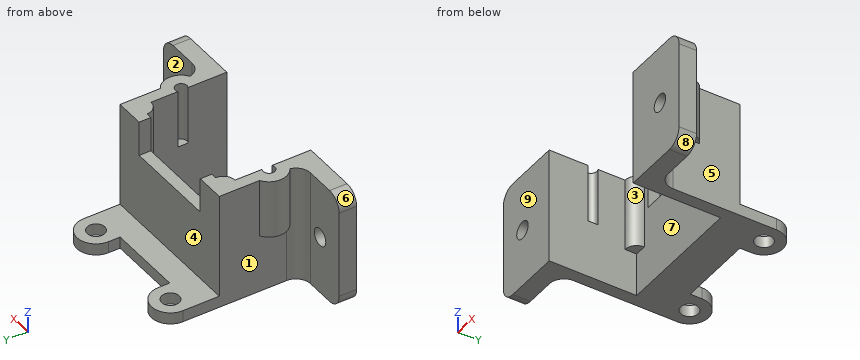
```python
from build123d import *

# Parameters (mm, degrees)
EXTRUDE_1_DEPTH     = 20
CUT_EXTRUDE_1_DEPTH = 20
EXTRUDE_2_DEPTH     = 12.5
SKETCH_4_W          = 4.208324297
SKETCH_4_H          = 5.852484321
SKETCH_4_W_2        = 6.809838445
SKETCH_4_H_2        = 5.603711631
CUT_EXTRUDE_2_DEPTH = 10
EXTRUDE_3_DEPTH     = 10
SKETCH_6_W          = 10
SKETCH_6_H          = 20
EXTRUDE_4_DEPTH     = 3
SKETCH_7_R          = 1.5
CUT_EXTRUDE_3_DEPTH = 3
FILLET_1_R          = 2.5
SKETCH_8_R          = 1.5
EXTRUDE_5_DEPTH     = 2


with BuildPart() as part:
    # 草图1 → 凸台-拉伸1 (new body)
    with BuildSketch(Plane.XY):
        with BuildLine():
            Line((-15.073529412, 6.665686275), (10.926470588, 6.665686275))
            Line((10.926470588, 6.665686275), (10.926470588, -0.236237514))
            ThreePointArc((10.926470588, -0.236237514), (12.426470588, -2.834313725), (10.926470588, -5.432389937))
            Line((10.926470588, -5.432389937), (10.926470588, -10.334313725))
            Line((10.926470588, -10.334313725), (8.926470588, -10.334313725))
            Line((8.926470588, -10.334313725), (8.926470588, -3.700339129))
            ThreePointArc((8.926470588, -3.700339129), (10.426470588, -2.834313725), (8.926470588, -1.968288322))
            Line((8.926470588, -1.968288322), (8.926470588, 4.665686275))
            Line((8.926470588, 4.665686275), (-13.073529412, 4.665686275))
            Line((-13.073529412, 4.665686275), (-13.073529412, -1.968288322))
            ThreePointArc((-13.073529412, -1.968288322), (-14.573529412, -2.834313725), (-13.073529412, -3.700339129))
            Line((-13.073529412, -3.700339129), (-13.073529412, -10.334313725))
            Line((-13.073529412, -10.334313725), (-15.073529412, -10.334313725))
            Line((-15.073529412, -10.334313725), (-15.073529412, -5.432389937))
            ThreePointArc((-15.073529412, -5.432389937), (-16.573529412, -2.834313725), (-15.073529412, -0.236237514))
            Line((-15.073529412, -0.236237514), (-15.073529412, 6.665686275))
        make_face()
    extrude(amount=EXTRUDE_1_DEPTH)

    # 草图2 → 切除-拉伸1 (cut)
    with BuildSketch(Plane(origin=(0, 6.665686275, 0), x_dir=(1, 0, 0), z_dir=(0, 1, 0))):
        Polygon((-2.073529412, -14), (-10.073529412, -14), (-10.073529412, -20), (5.926470588, -20), (5.926470588, -14), align=None)
    extrude(amount=-CUT_EXTRUDE_1_DEPTH, mode=Mode.SUBTRACT)

    # 草图3 → 凸台-拉伸2 (add)
    with BuildSketch(Plane.XY.offset(20)):
        with BuildLine():
            Line((-13.073529412, 4.665686275), (-13.073529412, 2.665686275))
            ThreePointArc((-13.073529412, 2.665686275), (-11.659315849, 3.251472712), (-11.073529412, 4.665686275))
            Line((-11.073529412, 4.665686275), (-13.073529412, 4.665686275))
        make_face()
        with BuildLine():
            Line((8.926470588, 4.665686275), (8.926470588, 2.665686275))
            ThreePointArc((8.926470588, 2.665686275), (7.512257026, 3.251472712), (6.926470588, 4.665686275))
            Line((6.926470588, 4.665686275), (8.926470588, 4.665686275))
        make_face()
    extrude(amount=-EXTRUDE_2_DEPTH)

    # 草图4 → 切除-拉伸2 (cut)
    with BuildSketch(Plane(origin=(0, 0, 0), x_dir=(-1, 0, 0), z_dir=(0, 0, -1))):
        with Locations((-13.030632737, -3.162479675)):
            Rectangle(SKETCH_4_W, SKETCH_4_H)
        with Locations((18.478448635, -3.03809333)):
            Rectangle(SKETCH_4_W_2, SKETCH_4_H_2)
    extrude(amount=-CUT_EXTRUDE_2_DEPTH, mode=Mode.SUBTRACT)

    # 草图5 → 凸台-拉伸3 (add)
    with BuildSketch(Plane(origin=(0, 0, 0), x_dir=(-1, 0, 0), z_dir=(0, 0, -1))):
        with BuildLine():
            Line((-8.926470588, -1.968288322), (-8.926470588, -3.700339129))
            ThreePointArc((-8.926470588, -3.700339129), (-10.426470588, -2.834313725), (-8.926470588, -1.968288322))
        make_face()
        with BuildLine():
            Line((13.073529412, -1.968288322), (13.073529412, -3.700339129))
            ThreePointArc((13.073529412, -3.700339129), (14.573529412, -2.834313725), (13.073529412, -1.968288322))
        make_face()
    extrude(amount=-EXTRUDE_3_DEPTH)

    # 草图6 → 凸台-拉伸4 (add)
    with BuildSketch(Plane.XZ.offset(10.334313725)):
        with Locations((15.926470588, 10)):
            Rectangle(SKETCH_6_W, SKETCH_6_H)
        with Locations((-20.073529412, 10)):
            Rectangle(SKETCH_6_W, SKETCH_6_H)
    extrude(amount=-EXTRUDE_4_DEPTH)

    # 草图7 → 切除-拉伸3 (cut)
    with BuildSketch(Plane(origin=(0, -7.334313725, 0), x_dir=(1, 0, 0), z_dir=(0, 1, 0))):
        with Locations(Location((15.926470588, -10, 0), (0, 0, 270))):
            Circle(SKETCH_7_R)
        with Locations(Location((-20.073529412, -10, 0), (0, 0, 270))):
            Circle(SKETCH_7_R)
    extrude(amount=-CUT_EXTRUDE_3_DEPTH, mode=Mode.SUBTRACT)

    # 圆角1
    fillet_1_edges = [part.edges().sort_by_distance(p)[0] for p in [
        (-15.073529412, -7.334313725, 10),
        (10.926470588, -7.334313725, 10),
        (20.926470588, -8.834313725, 20),
        (-25.073529412, -8.834313725, 20),
        (20.926470588, -8.834313725, 0),
        (-25.073529412, -8.834313725, 0),
    ]]
    fillet(fillet_1_edges, radius=FILLET_1_R)

    # 草图8 → 凸台-拉伸5 (add)
    with BuildSketch(Plane(origin=(0, 0, 0), x_dir=(-1, 0, 0), z_dir=(0, 0, -1))):
        with BuildLine():
            Line((-4.426470588, 10.915686275), (8.573529412, 10.915686275))
            Line((8.573529412, 10.915686275), (8.573529412, 12.915686275))
            ThreePointArc((8.573529412, 12.915686275), (11.823529412, 16.165686275), (15.073529412, 12.915686275))
            Line((15.073529412, 12.915686275), (15.073529412, 6.665686275))
            Line((15.073529412, 6.665686275), (8.573529412, 6.665686275))
            Line((8.573529412, 6.665686275), (-4.426470588, 6.665686275))
            Line((-4.426470588, 6.665686275), (-10.926470588, 6.665686275))
            Line((-10.926470588, 6.665686275), (-10.926470588, 12.915686275))
            ThreePointArc((-10.926470588, 12.915686275), (-7.676470588, 16.165686275), (-4.426470588, 12.915686275))
            Line((-4.426470588, 12.915686275), (-4.426470588, 10.915686275))
        make_face()
        with Locations((-7.676470588, 12.915686275)):
            Circle(SKETCH_8_R, mode=Mode.SUBTRACT)
        with Locations((11.823529412, 12.915686275)):
            Circle(SKETCH_8_R, mode=Mode.SUBTRACT)
    extrude(amount=-EXTRUDE_5_DEPTH)


solid = part.part
```
For this review, take the finished solid that the model builds, in its own axes (mm). Face numbers are marked on the shaded views. A direction names the side the tool comes from. Coordinates: 2 decimals unless noted, no trailing zeros. Write each loop counter-clockwise with the first axis right and the second up, starting at its lowest first coordinate (ties: lowest second). Pieces come first, ordered by that corner, then holes. Notation, with made-up numbers: (7, 70) - (62, 70) arc R32 cw to (62, 104) - close; hole circle Ø5 at (41, 58). An arc over 180 degrees is marked (long way). Answer in a Markdown table with one row per item. Add a question column.
Q1. Tool access review of the marked faces 1, 2, 3, 4 and 5: name each direction out of +Z, -Z, +X, -X, +Y, -Y from which nothing blocks a thin tool from reaching the whole face with its end or side.
Q2. For probe 1 along X at (y, z) = (-8.45, 10); probe 2 along X at (y, z) = (-3, 1.25); probe 3 along X at (y, z) = (5.5, 1.75), list the stretches that pass through material, from the lowest coordinate up.
Q3. Draft analysis for pull direction X (two halves, no side actions). For the marked faces 6, 7, 8 and 9, state which applies: +X half, -X half, draft (parallel to the pull), parting line (faces both ways), or undercut.
Q4. We need section B-B, the plane z = 11. Count the separate pieces of the cut face and the enclosed holes in it, and give its area (3 significant figures).
Q5. For P1, Ø1.8, axis at x = 9.43, y = -2.83, coming from the +Z side; P2, Ø1, axis at y = 12, z = 1.5, coming from the +X side; P3, Ø2, axis at x = 18, z = 10, coming from the +Y side, all flat-tipped, find the tip position at first contact; note any pin that passes through.
Q6. We need section A-A, the plane y = 0.5. State the section outline as (x, z) points.
Q7. We need section C-C, the plane y = 5.5. State the section outline as (x, z) points, and give its area (3 significant figures).
Q8. We need section D-D, the plane z = 14.5. State the section outline as (x, y) points, and give its area (3 significant figures).
Answer list:
| question | item | result |
|---|---|---|
| 1 | face 1 | -Z, -X, +Y |
| 1 | face 2 | +Z, -Z, +X, +Y |
| 1 | face 3 | +Z, -Z, -Y |
| 1 | face 4 | +Z, +X, -X, +Y |
| 1 | face 5 | -Z, +X, +Y |
| 2 | probe 1 | x = -25.07 to -21.57, -18.57 to -13.07, 8.93 to 14.43, 17.43 to 20.93 |
| 2 | probe 2 | x = -15.07 to -13.07, 8.93 to 10.93 |
| 2 | probe 3 | x = -15.07 to 10.93 |
| 3 | face 6 | -X half |
| 3 | face 7 | undercut |
| 3 | face 8 | +X half |
| 3 | face 9 | draft |
| 4 | separate pieces | 3 |
| 4 | enclosed holes | 0 |
| 4 | area | 174 mm2 |
| 5 | P1 | stops at z = 10 |
| 5 | P2 | stops at x = 10.93 |
| 5 | P3 | stops at y = -7.33 |
| 6 | outline | (-15.07, 0) - (-13.07, 0) - (-13.07, 20) - (-15.07, 20) - close; (8.93, 0) - (10.93, 0) - (10.93, 20) - (8.93, 20) - close |
| 7 | outline | (-15.07, 0) - (10.93, 0) - (10.93, 20) - (5.93, 20) - (5.93, 14) - (-10.07, 14) - (-10.07, 20) - (-15.07, 20) - close |
| 7 | area | 424 mm2 |
| 8 | outline | (-25.07, -10.33) - (-13.07, -10.33) - (-13.07, -3.7) arc R1 cw (long way) to (-13.07, -1.97) - (-13.07, 2.67) arc R2 ccw to (-11.07, 4.67) - (-10.07, 4.67) - (-10.07, 6.67) - (-15.07, 6.67) - (-15.07, -0.24) arc R3 ccw to (-15.14, -5.39) arc R2.5 cw to (-17.57, -7.33) - (-25.07, -7.33) - close; (5.93, 4.67) - (6.93, 4.67) arc R2 ccw to (8.93, 2.67) - (8.93, -1.97) arc R1 cw (long way) to (8.93, -3.7) - (8.93, -10.33) - (20.93, -10.33) - (20.93, -7.33) - (13.43, -7.33) arc R2.5 cw to (10.99, -5.39) arc R3 ccw to (10.93, -0.24) - (10.93, 6.67) - (5.93, 6.67) - close |
| 8 | area | 155 mm2 |
